```python
from build123d import *

# Parameters (mm, degrees)
BOSS_EXTRUDE1_DEPTH         = 5
FILLET3_RADIUS              = 10
FILLET3_LENGTH              = 5
FILLET4_RADIUS              = 10
FILLET4_LENGTH              = 5
FILLET2_R                   = 2
SKETCH2_R                   = 1.6
LAYER_FIX_HOLE_DEPTH        = 213.55881539
CHAMFER1_SIZE               = 3
MOTOR_FIX_HOLE_REACH        = 214.559
SKETCH9_R                   = 4
MOTOR_DRIVER_FIX_HOLE_REACH = 214.559
SKETCH10_R                  = 1.75
SKETCH11_R                  = 1
SKETCH11_W                  = 20
SKETCH11_H                  = 5
QTR8A_FIX_HOLE_DEPTH        = 10
SKETCH_12_W                 = 5
SKETCH_12_H                 = 10
BATTERY_FIXED_HOLE_DEPTH    = 213.55881539


with BuildPart() as part:
    # Sketch1 → Boss-Extrude1 (new body)
    with BuildSketch(Plane(origin=(0, 0, 0), x_dir=(1, 0, 0), z_dir=(0, 1, 0))):
        Polygon((-117.5, -130), (117.5, -130), (117.5, -110), (107.5, -110), (107.5, -40), (117.5, -40), (117.5, 80), (107.5, 80), (107.5, 150), (127.5, 150), (127.5, 170), (-127.5, 170), (-127.5, 150), (-107.5, 150), (-107.5, 80), (-117.5, 80), (-117.5, -40), (-107.5, -40), (-107.5, -110), (-117.5, -110), align=None)
    extrude(amount=BOSS_EXTRUDE1_DEPTH)

    # Fillet3: full round fillet: the end face becomes a half cylinder, R = half its width
    fillet3_face = Plane((127.5, 2.5, -160), x_dir=(0, 1, 0), z_dir=(1, 0, 0))  # on the end face: x along it, z out of the body
    fillet3_slab = fillet3_face.offset(-FILLET3_RADIUS / 2) * Box(FILLET3_LENGTH, 2 * FILLET3_RADIUS, FILLET3_RADIUS, mode=Mode.PRIVATE)  # the body's end, R deep
    fillet3_round = Plane((117.5, 2.5, -160), x_dir=(1, 0, 0), z_dir=(0, 1, 0)) * Cylinder(FILLET3_RADIUS, FILLET3_LENGTH, mode=Mode.PRIVATE)  # its axis R under the face
    add(fillet3_slab - fillet3_round, mode=Mode.SUBTRACT)

    # Fillet4: full round fillet: the end face becomes a half cylinder, R = half its width
    fillet4_face = Plane((-127.5, 2.5, -160), x_dir=(0, 1, 0), z_dir=(-1, 0, 0))  # on the end face: x along it, z out of the body
    fillet4_slab = fillet4_face.offset(-FILLET4_RADIUS / 2) * Box(FILLET4_LENGTH, 2 * FILLET4_RADIUS, FILLET4_RADIUS, mode=Mode.PRIVATE)  # the body's end, R deep
    fillet4_round = Plane((-117.5, 2.5, -160), x_dir=(-1, 0, 0), z_dir=(0, 1, 0)) * Cylinder(FILLET4_RADIUS, FILLET4_LENGTH, mode=Mode.PRIVATE)  # its axis R under the face
    add(fillet4_slab - fillet4_round, mode=Mode.SUBTRACT)

    # Fillet2
    fillet2_edges = [part.edges().sort_by_distance(p)[0] for p in [
        (117.5, 2.5, 130),
        (-117.5, 2.5, 130),
        (-107.5, 2.5, 110),
        (-107.5, 2.5, 40),
        (-107.5, 2.5, -80),
        (-107.5, 2.5, -150),
        (107.5, 2.5, -150),
        (107.5, 2.5, -80),
        (107.5, 2.5, 40),
        (107.5, 2.5, 110),
    ]]
    fillet(fillet2_edges, radius=FILLET2_R)

    # Sketch2 → layer fix hole (cut, through all)
    with BuildSketch(Plane(origin=(0, 5, 0), x_dir=(1, 0, 0), z_dir=(0, 1, 0))):
        with Locations(Location((107.5, 160, 0), (0, 0, 270))):
            Circle(SKETCH2_R)
        with Locations(Location((107.5, 20, 0), (0, 0, 270))):
            Circle(SKETCH2_R)
        with Locations(Location((107.5, -119, 0), (0, 0, 270))):
            Circle(SKETCH2_R)
        with Locations(Location((0, -119, 0), (0, 0, 90))):
            Circle(SKETCH2_R)
        with Locations(Location((-107.5, -119, 0), (0, 0, 90))):
            Circle(SKETCH2_R)
        with Locations(Location((-107.5, 20, 0), (0, 0, 90))):
            Circle(SKETCH2_R)
        with Locations(Location((-107.5, 160, 0), (0, 0, 90))):
            Circle(SKETCH2_R)
        with Locations(Location((55, -119, 0), (0, 0, 90))):
            Circle(SKETCH2_R)
        with Locations(Location((-55, -119, 0), (0, 0, 90))):
            Circle(SKETCH2_R)
        with Locations(Location((-107.5, 70, 0), (0, 0, 90))):
            Circle(SKETCH2_R)
        with Locations(Location((107.5, 70, 0), (0, 0, 270))):
            Circle(SKETCH2_R)
        with Locations(Location((-107.5, -30, 0), (0, 0, 90))):
            Circle(SKETCH2_R)
        with Locations(Location((107.5, -30, 0), (0, 0, 270))):
            Circle(SKETCH2_R)
    extrude(amount=-LAYER_FIX_HOLE_DEPTH, mode=Mode.SUBTRACT)

    # Chamfer1
    chamfer1_edges = [part.edges().sort_by_distance(p)[0] for p in [
        (-117.5, 2.5, 110),
        (-117.5, 2.5, 40),
        (-117.5, 2.5, -80),
        (117.5, 2.5, -80),
        (117.5, 2.5, 40),
        (117.5, 2.5, 110),
    ]]
    chamfer(chamfer1_edges, length=CHAMFER1_SIZE)

    # Sketch9 → Motor fix hole (cut, up to next)
    with BuildSketch(Plane.XZ, mode=Mode.PRIVATE) as motor_fix_hole_sk1:
        with Locations(Location((-80.5, -138, 0), (0, 0, 270))):
            Circle(SKETCH9_R)
    motor_fix_hole_tool1 = extrude(motor_fix_hole_sk1.sketch, amount=-MOTOR_FIX_HOLE_REACH, mode=Mode.PRIVATE) & part.part
    # Sketch9 → Motor fix hole (cut, up to next)
    with BuildSketch(Plane.XZ, mode=Mode.PRIVATE) as motor_fix_hole_sk2:
        with Locations(Location((-80.5, -92, 0), (0, 0, 90))):
            Circle(SKETCH9_R)
    motor_fix_hole_tool2 = extrude(motor_fix_hole_sk2.sketch, amount=-MOTOR_FIX_HOLE_REACH, mode=Mode.PRIVATE) & part.part
    # Sketch9 → Motor fix hole (cut, up to next)
    with BuildSketch(Plane.XZ, mode=Mode.PRIVATE) as motor_fix_hole_sk3:
        with Locations(Location((80.5, -92, 0), (0, 0, 270))):
            Circle(SKETCH9_R)
    motor_fix_hole_tool3 = extrude(motor_fix_hole_sk3.sketch, amount=-MOTOR_FIX_HOLE_REACH, mode=Mode.PRIVATE) & part.part
    # Sketch9 → Motor fix hole (cut, up to next)
    with BuildSketch(Plane.XZ, mode=Mode.PRIVATE) as motor_fix_hole_sk4:
        with Locations(Location((80.5, -138, 0), (0, 0, 90))):
            Circle(SKETCH9_R)
    motor_fix_hole_tool4 = extrude(motor_fix_hole_sk4.sketch, amount=-MOTOR_FIX_HOLE_REACH, mode=Mode.PRIVATE) & part.part
    # Sketch9 → Motor fix hole (cut, up to next)
    with BuildSketch(Plane.XZ, mode=Mode.PRIVATE) as motor_fix_hole_sk5:
        with Locations(Location((80.5, 98, 0), (0, 0, 270))):
            Circle(SKETCH9_R)
    motor_fix_hole_tool5 = extrude(motor_fix_hole_sk5.sketch, amount=-MOTOR_FIX_HOLE_REACH, mode=Mode.PRIVATE) & part.part
    # Sketch9 → Motor fix hole (cut, up to next)
    with BuildSketch(Plane.XZ, mode=Mode.PRIVATE) as motor_fix_hole_sk6:
        with Locations(Location((80.5, 52, 0), (0, 0, 90))):
            Circle(SKETCH9_R)
    motor_fix_hole_tool6 = extrude(motor_fix_hole_sk6.sketch, amount=-MOTOR_FIX_HOLE_REACH, mode=Mode.PRIVATE) & part.part
    # Sketch9 → Motor fix hole (cut, up to next)
    with BuildSketch(Plane.XZ, mode=Mode.PRIVATE) as motor_fix_hole_sk7:
        with Locations(Location((-80.5, 98, 0), (0, 0, 90))):
            Circle(SKETCH9_R)
    motor_fix_hole_tool7 = extrude(motor_fix_hole_sk7.sketch, amount=-MOTOR_FIX_HOLE_REACH, mode=Mode.PRIVATE) & part.part
    # Sketch9 → Motor fix hole (cut, up to next)
    with BuildSketch(Plane.XZ, mode=Mode.PRIVATE) as motor_fix_hole_sk8:
        with Locations(Location((-80.5, 52, 0), (0, 0, 270))):
            Circle(SKETCH9_R)
    motor_fix_hole_tool8 = extrude(motor_fix_hole_sk8.sketch, amount=-MOTOR_FIX_HOLE_REACH, mode=Mode.PRIVATE) & part.part
    add(motor_fix_hole_tool1.solids().sort_by_distance((-80.5, 0, -138))[0], mode=Mode.SUBTRACT)
    add(motor_fix_hole_tool2.solids().sort_by_distance((-80.5, 0, -92))[0], mode=Mode.SUBTRACT)
    add(motor_fix_hole_tool3.solids().sort_by_distance((80.5, 0, -92))[0], mode=Mode.SUBTRACT)
    add(motor_fix_hole_tool4.solids().sort_by_distance((80.5, 0, -138))[0], mode=Mode.SUBTRACT)
    add(motor_fix_hole_tool5.solids().sort_by_distance((80.5, 0, 98))[0], mode=Mode.SUBTRACT)
    add(motor_fix_hole_tool6.solids().sort_by_distance((80.5, 0, 52))[0], mode=Mode.SUBTRACT)
    add(motor_fix_hole_tool7.solids().sort_by_distance((-80.5, 0, 98))[0], mode=Mode.SUBTRACT)
    add(motor_fix_hole_tool8.solids().sort_by_distance((-80.5, 0, 52))[0], mode=Mode.SUBTRACT)

    # Sketch10 → Motor driver fix hole (cut, up to next)
    with BuildSketch(Plane.XZ, mode=Mode.PRIVATE) as motor_driver_fix_hole_sk1:
        with Locations(Location((18.68975044, 75, 0), (0, 0, 270))):
            Circle(SKETCH10_R)
    motor_driver_fix_hole_tool1 = extrude(motor_driver_fix_hole_sk1.sketch, amount=-MOTOR_DRIVER_FIX_HOLE_REACH, mode=Mode.PRIVATE) & part.part
    # Sketch10 → Motor driver fix hole (cut, up to next)
    with BuildSketch(Plane.XZ, mode=Mode.PRIVATE) as motor_driver_fix_hole_sk2:
        with Locations(Location((-18.68975044, 75, 0), (0, 0, 270))):
            Circle(SKETCH10_R)
    motor_driver_fix_hole_tool2 = extrude(motor_driver_fix_hole_sk2.sketch, amount=-MOTOR_DRIVER_FIX_HOLE_REACH, mode=Mode.PRIVATE) & part.part
    # Sketch10 → Motor driver fix hole (cut, up to next)
    with BuildSketch(Plane.XZ, mode=Mode.PRIVATE) as motor_driver_fix_hole_sk3:
        with Locations(Location((-18.68975044, 111.74180032, 0), (0, 0, 270))):
            Circle(SKETCH10_R)
    motor_driver_fix_hole_tool3 = extrude(motor_driver_fix_hole_sk3.sketch, amount=-MOTOR_DRIVER_FIX_HOLE_REACH, mode=Mode.PRIVATE) & part.part
    # Sketch10 → Motor driver fix hole (cut, up to next)
    with BuildSketch(Plane.XZ, mode=Mode.PRIVATE) as motor_driver_fix_hole_sk4:
        with Locations(Location((18.68975044, 111.74180032, 0), (0, 0, 270))):
            Circle(SKETCH10_R)
    motor_driver_fix_hole_tool4 = extrude(motor_driver_fix_hole_sk4.sketch, amount=-MOTOR_DRIVER_FIX_HOLE_REACH, mode=Mode.PRIVATE) & part.part
    # Sketch10 → Motor driver fix hole (cut, up to next)
    with BuildSketch(Plane.XZ, mode=Mode.PRIVATE) as motor_driver_fix_hole_sk5:
        with Locations(Location((18.68975044, -151.74180032, 0), (0, 0, 90))):
            Circle(SKETCH10_R)
    motor_driver_fix_hole_tool5 = extrude(motor_driver_fix_hole_sk5.sketch, amount=-MOTOR_DRIVER_FIX_HOLE_REACH, mode=Mode.PRIVATE) & part.part
    # Sketch10 → Motor driver fix hole (cut, up to next)
    with BuildSketch(Plane.XZ, mode=Mode.PRIVATE) as motor_driver_fix_hole_sk6:
        with Locations(Location((-18.68975044, -151.74180032, 0), (0, 0, 90))):
            Circle(SKETCH10_R)
    motor_driver_fix_hole_tool6 = extrude(motor_driver_fix_hole_sk6.sketch, amount=-MOTOR_DRIVER_FIX_HOLE_REACH, mode=Mode.PRIVATE) & part.part
    # Sketch10 → Motor driver fix hole (cut, up to next)
    with BuildSketch(Plane.XZ, mode=Mode.PRIVATE) as motor_driver_fix_hole_sk7:
        with Locations(Location((-18.68975044, -115, 0), (0, 0, 90))):
            Circle(SKETCH10_R)
    motor_driver_fix_hole_tool7 = extrude(motor_driver_fix_hole_sk7.sketch, amount=-MOTOR_DRIVER_FIX_HOLE_REACH, mode=Mode.PRIVATE) & part.part
    # Sketch10 → Motor driver fix hole (cut, up to next)
    with BuildSketch(Plane.XZ, mode=Mode.PRIVATE) as motor_driver_fix_hole_sk8:
        with Locations(Location((18.68975044, -115, 0), (0, 0, 90))):
            Circle(SKETCH10_R)
    motor_driver_fix_hole_tool8 = extrude(motor_driver_fix_hole_sk8.sketch, amount=-MOTOR_DRIVER_FIX_HOLE_REACH, mode=Mode.PRIVATE) & part.part
    add(motor_driver_fix_hole_tool1.solids().sort_by_distance((18.68975, 0, 75))[0], mode=Mode.SUBTRACT)
    add(motor_driver_fix_hole_tool2.solids().sort_by_distance((-18.68975, 0, 75))[0], mode=Mode.SUBTRACT)
    add(motor_driver_fix_hole_tool3.solids().sort_by_distance((-18.68975, 0, 111.7418))[0], mode=Mode.SUBTRACT)
    add(motor_driver_fix_hole_tool4.solids().sort_by_distance((18.68975, 0, 111.7418))[0], mode=Mode.SUBTRACT)
    add(motor_driver_fix_hole_tool5.solids().sort_by_distance((18.68975, 0, -151.7418))[0], mode=Mode.SUBTRACT)
    add(motor_driver_fix_hole_tool6.solids().sort_by_distance((-18.68975, 0, -151.7418))[0], mode=Mode.SUBTRACT)
    add(motor_driver_fix_hole_tool7.solids().sort_by_distance((-18.68975, 0, -115))[0], mode=Mode.SUBTRACT)
    add(motor_driver_fix_hole_tool8.solids().sort_by_distance((18.68975, 0, -115))[0], mode=Mode.SUBTRACT)

    # Sketch11 → QTR8a fix hole (cut)
    with BuildSketch(Plane.XZ):
        with Locations(Location((-34.737301465, -159, 0), (0, 0, 270))):
            Circle(SKETCH11_R)
        with Locations(Location((-21.513799845, -159, 0), (0, 0, 270))):
            Circle(SKETCH11_R)
        with Locations(Location((-16.814799845, -159, 0), (0, 0, 270))):
            Circle(SKETCH11_R)
        with Locations(Location((34.737301775, -159, 0), (0, 0, 270))):
            Circle(SKETCH11_R)
        with Locations((0, -146.5)):
            Rectangle(SKETCH11_W, SKETCH11_H)
    extrude(amount=-QTR8A_FIX_HOLE_DEPTH, mode=Mode.SUBTRACT)

    # Sketch 12 → Battery fixed hole (cut, through all)
    with BuildSketch(Plane(origin=(0, 5, 0), x_dir=(1, 0, 0), z_dir=(0, 1, 0))):
        with Locations((26.666666667, 55)):
            Rectangle(SKETCH_12_W, SKETCH_12_H)
        with Locations((101.666666667, 55)):
            Rectangle(SKETCH_12_W, SKETCH_12_H)
        with Locations((26.666666667, -15)):
            Rectangle(SKETCH_12_W, SKETCH_12_H)
        with Locations((101.666666667, -15)):
            Rectangle(SKETCH_12_W, SKETCH_12_H)
        with Locations((-101.666666667, 55)):
            Rectangle(SKETCH_12_W, SKETCH_12_H)
        with Locations((-26.666666667, 55)):
            Rectangle(SKETCH_12_W, SKETCH_12_H)
        with Locations((-101.666666667, -15)):
            Rectangle(SKETCH_12_W, SKETCH_12_H)
        with Locations((-26.666666667, -15)):
            Rectangle(SKETCH_12_W, SKETCH_12_H)
    extrude(amount=-BATTERY_FIXED_HOLE_DEPTH, mode=Mode.SUBTRACT)


solid = part.part
```
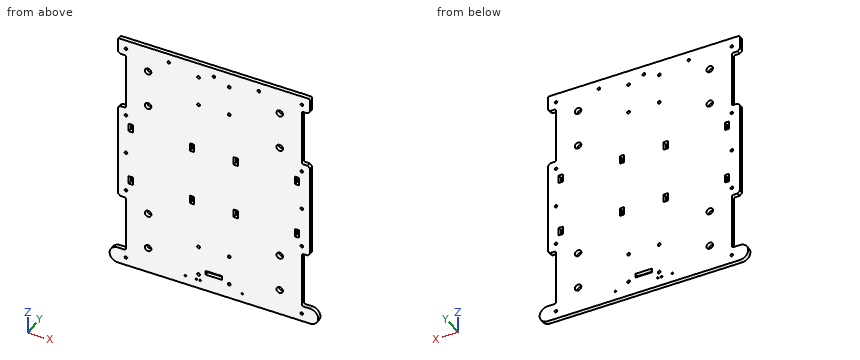
CAD build for the part. Positions are in the model's coordinates, mm. Coordinates: 2 decimals unless noted, no trailing zeros. Write each loop counter-clockwise with the first axis right and the second up, starting at its lowest first coordinate (ties: lowest second). Pieces come first, ordered by that corner, then holes. Notation, with made-up numbers: (9.25, 55.25) -> (15.25, 55.25) arc R30 ccw to (15.25, 83.25) -> close; hole circle Ø2 at (41, 53.25). An arc over 180 degrees is marked (long way). Return JSON: item names as keys, results as strings. Group by question number.
Q1. Cut at B-B, the plane z = 66. Give the cut face in (x, y), then the cut area to 4 significant figures.
Q2. Cut at A-A, the plane z = -92. Give the cut face in (x, y).
Q3. Drill centre lines: line 1 (X direction, y = 3.1, z = 52); line 2 (X direction, y = 3.75, z = 119); line 3 (Z direction, x = 5.5, y = 1.75). Where is each one in solid material? Low to high.
Q4. Cut at C-C, the plane y = 2.25. State how many separate pieces and enclosed holes the cut face has, then the cut area to 3 significant figures.
Q5. Flat gauge pins, fed straight in: pin 1 (2.5 mm diameter, centred on y = 2, z = 13, fed in from +X); pin 2 (1.5 mm diameter, centred on y = 2.5, z = -106, fed in from +X). Where does each tip first touch, or does it go through?
Returned:
{
 "1": {"outline": "(-107.5, 0) -> (107.5, 0) -> (107.5, 5) -> (-107.5, 5) -> close", "area": "1,075 mm2"},
 "2": {"outline": "(-107.5, 0) -> (-84.5, 0) -> (-84.5, 5) -> (-107.5, 5) -> close; (-76.5, 0) -> (76.5, 0) -> (76.5, 5) -> (-76.5, 5) -> close; (84.5, 0) -> (107.5, 0) -> (107.5, 5) -> (84.5, 5) -> close"},
 "3": {"line 1": "x = -107.5 to -84.5, -76.5 to 76.5, 84.5 to 107.5", "line 2": "x = -117.5 to -109.1, -105.9 to -56.6, -53.4 to -1.6, 1.6 to 53.4, 56.6 to 105.9, 109.1 to 117.5", "line 3": "z = -170 to -149, -144 to 130"},
 "4": {"separate pieces": "1", "enclosed holes": "42", "area": "66,900 mm2"},
 "5": {"pin 1": "stops at x = 117.5", "pin 2": "stops at x = 107.5"}
}
